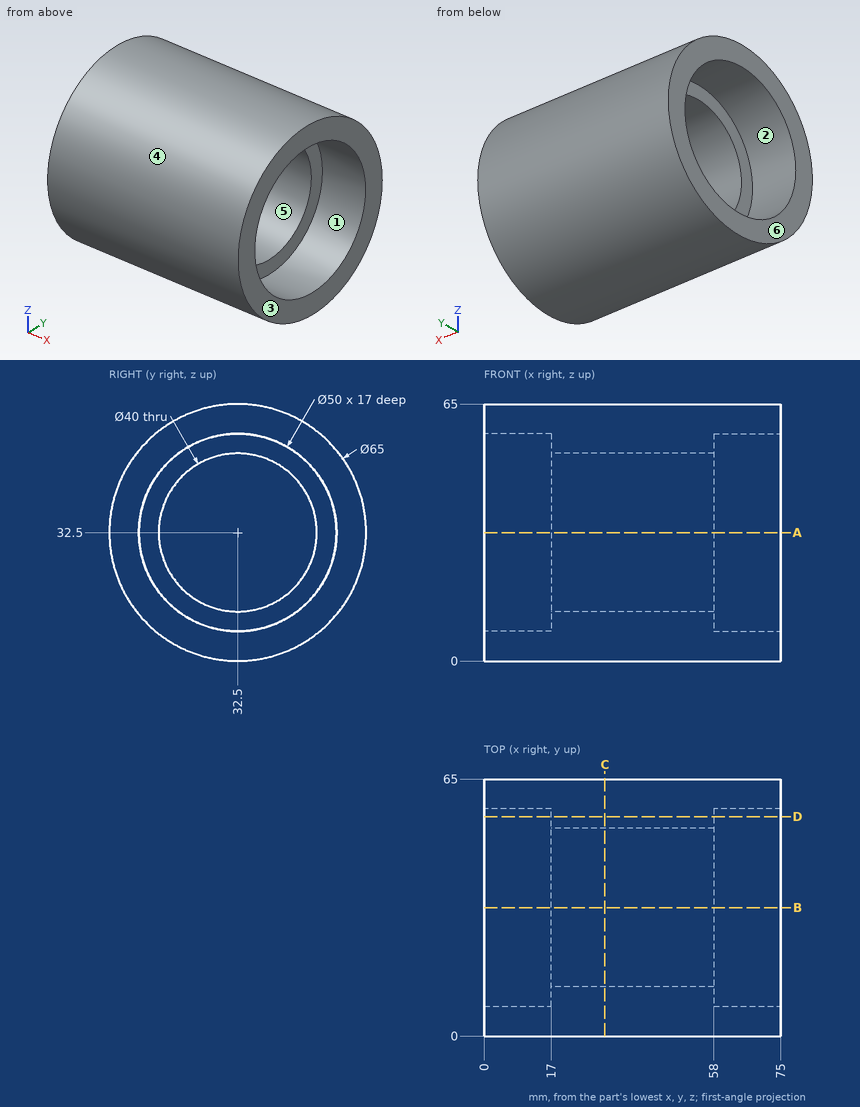
Print and shaded views of the part. All mm, measured from the part's lowest x, y and z. A direction names the side the tool comes from. Coordinates: 2 decimals unless noted, no trailing zeros. Order: outer loops, then holes, each group sorted by start corner. A loop starts at its lowest first (then second) coordinate and runs counter-clockwise, first axis right, second up. Notation, with made-up numbers: M 69,45 L 109,45 A28 ccw 109,63 Z; hole C 29,53 d6. An arc over 180 degrees is marked long. Answer as CSV lines item,"result".
1) Cut at D-D (y = 55.5). List the corners of the cut face in (x, z), then the cut area to 3 significant figures.
Verdict:
outline,"M 0,9.54 L 75,9.54 L 75,22.7 L 58,22.7 L 58,42.3 L 75,42.3 L 75,55.46 L 0,55.46 L 0,42.3 L 17,42.3 L 17,22.7 L 0,22.7 Z"
area,"2,780 mm2"
2) Cut at C-C (x = 30.5). List the corners of the cut face in (y, z), then the cut area to 3 significant figures.
Verdict:
outline,"C 32.5,32.5 d65; hole C 32.5,32.5 d40"
area,"2,060 mm2"
3) Flat gauge pins, fed straight in: P1, Ø1.5, axis at x = 47, z = 49, coming from the +Y side; P2, Ø5, axis at x = 46, y = 21.5, coming from the +Z side; P3, Ø1, axis at x = 45, z = 48, coming from the -Y side; P4, Ø6, axis at y = 47, z = 58, coming from the -X side. Where does each tip first touch, or does it go through?
Verdict:
P1,"y = 60.93"
P2,"z = 63.87"
P3,"y = 3.67"
P4,"x = 0"
4) 3-axis set-ups, long thin cutter, end or side, ignore diameter. For the marked faces 1, 2 and 3: which of +Z, -Z, +X, -X, +Y, -Y reach the whole face in a straight line?
Verdict:
face 1,"+X"
face 2,"-X"
face 3,"+Z, -Z, +X, +Y, -Y"
5) Mould opens along Y. For the marked faces 4, 5 and 6 say: released by +Y, released by -Y, zero draft, split by the parting line, or undercut.
Verdict:
face 4,"split by the parting line"
face 5,"undercut"
face 6,"zero draft"
6) Drill centre lines: L1, parallel to Y at x = 42, z = 32; L2, parallel to Z at x = 66, y = 32 (3 decimals). Where is each one in solid material? Low to high. Write a range as from..to.
Verdict:
L1,"0..12.51, 52.49..65"
L2,"0.004..7.505, 57.495..64.996"
7) Cut at A-A (z = 32.5). List the corners of the cut face in (x, y).
Verdict:
outline,"M 0,0 L 75,0 L 75,7.5 L 58,7.5 L 58,12.5 L 17,12.5 L 17,7.5 L 0,7.5 Z; M 0,57.5 L 17,57.5 L 17,52.5 L 58,52.5 L 58,57.5 L 75,57.5 L 75,65 L 0,65 Z"
